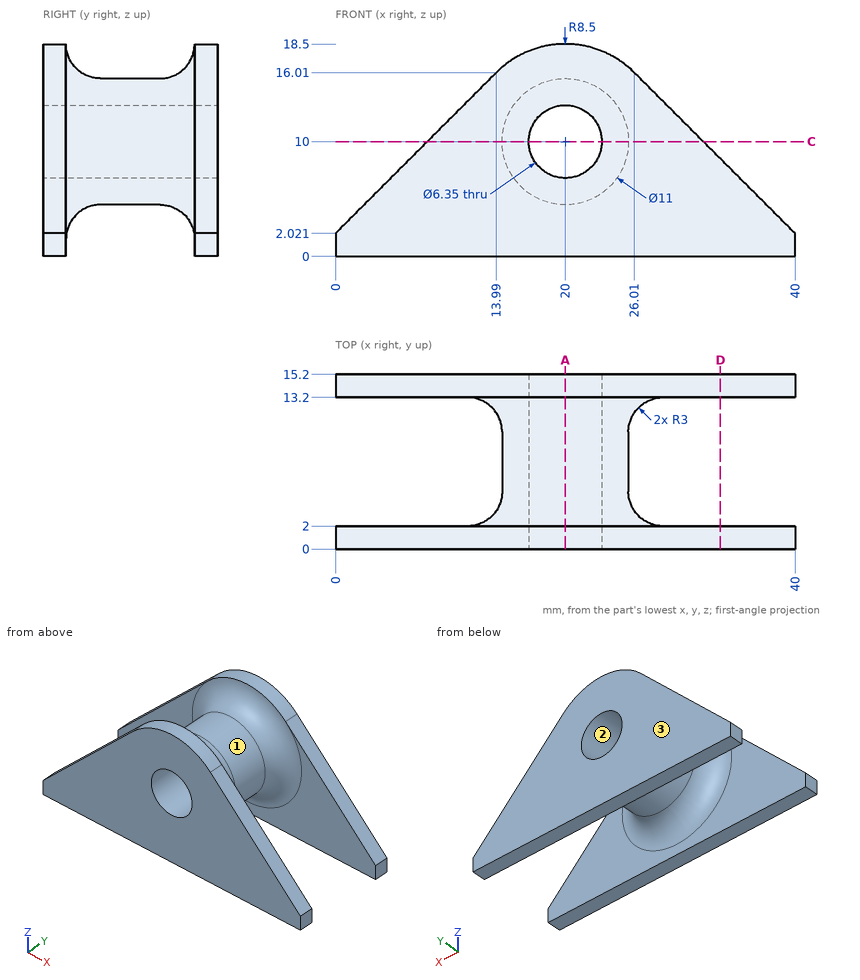
Input: dimensioned drawing with shaded views. Units: mm. Origin: part minimum x, y, z. Coordinates: 2 decimals unless noted, no trailing zeros. Order: outer loops, then holes, each group sorted by start corner. A loop starts at its lowest first (then second) coordinate and runs counter-clockwise, first axis right, second up. Notation, with made-up numbers: (65, 22.5) - (106, 22.5) arc R24 ccw to (106, 47.5) - close; hole circle Ø5 at (-21, -18.75). An arc over 180 degrees is marked (long way). One line per item, written item: value.
1) Mould query, pull axis Z, two halves, no side actions, for the marked faces 1, 2 and 3. Classes: released by +Z, released by -Z, zero draft, split by the parting line, or undercut.
Computed values:
face 1: split by the parting line
face 2: undercut
face 3: zero draft
2) Ray query, line 1 (Y direction, x = 23.5, z = 17.5); line 2 (X direction, y = 7.75, z = 10) (1 decimal); line 3 (Y direction, x = 16.5, z = 17). Return the intervals inside material, ascending. Write a range as [from, to].
Computed values:
line 1: y = [0, 2.01], [13.19, 15.2]
line 2: x = [14.5, 16.8], [23.2, 25.5]
line 3: y = [0, 2.08], [13.12, 15.2]
3) Cut plane D-D on x = 33.5. Output: boundary loops of the cut face in (y, z).
Computed values:
outline: (0, 0) - (2, 0) - (2, 8.52) - (0, 8.52) - close; (13.2, 0) - (15.2, 0) - (15.2, 8.52) - (13.2, 8.52) - close
4) Cut plane C-C on z = 10. Output: boundary loops of the cut face in (x, y) (1 decimal).
Computed values:
outline: (8, 0) - (16.8, 0) - (16.8, 15.2) - (8, 15.2) - (8, 13.2) - (11.5, 13.2) arc R3 cw to (14.5, 10.2) - (14.5, 5) arc R3 cw to (11.5, 2) - (8, 2) - close; (23.2, 0) - (32, 0) - (32, 2) - (28.5, 2) arc R3 cw to (25.5, 5) - (25.5, 10.2) arc R3 cw to (28.5, 13.2) - (32, 13.2) - (32, 15.2) - (23.2, 15.2) - close
5) Contact query for a flat-ended pin moving along its axis: pin 1 (3 mm diameter, centred on y = 9.5, z = 6, fed in from +X). Output: stop coordinate, or through.
Computed values:
pin 1: stops at x = 24.9
6) Cut plane A-A on x = 20. Output: boundary loops of the cut face in (y, z) (1 decimal).
Computed values:
outline: (0, 0) - (2, 0) - (2, 1.5) arc R3 cw to (5, 4.5) - (10.2, 4.5) arc R3 cw to (13.2, 1.5) - (13.2, 0) - (15.2, 0) - (15.2, 6.8) - (0, 6.8) - close; (0, 13.2) - (15.2, 13.2) - (15.2, 18.5) - (13.2, 18.5) arc R3 cw to (10.2, 15.5) - (5, 15.5) arc R3 cw to (2, 18.5) - (0, 18.5) - close
